```python
from build123d import *

# Parameters (mm, degrees)
F0_R     = 50
F1_DEPTH = 35
F2_R     = 25
F3_DEPTH = 35
F4_R     = 7
F5_DEPTH = 50.001


with BuildPart() as f1:
    # F0 (on Top) → F1 (new body)
    with BuildSketch(Plane.XY):
        Circle(F0_R)
    extrude(amount=F1_DEPTH)

    # F2 (on Top) → F3 (cut)
    with BuildSketch(Plane.XY):
        Circle(F2_R)
    extrude(amount=F3_DEPTH, mode=Mode.SUBTRACT)

    # F4 (on Right) → F5 (cut, through all)
    with BuildSketch(Plane.YZ):
        Circle(F4_R)
    extrude(amount=F5_DEPTH, mode=Mode.SUBTRACT)


solid = f1.part
```
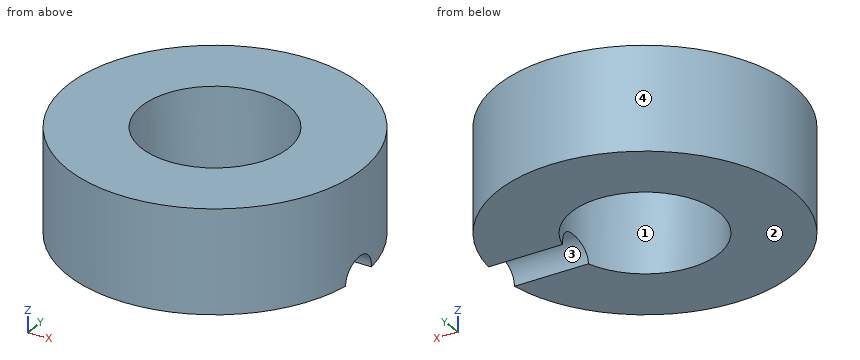
Build history of the part. All positions in model axes, mm. Face numbers are marked on the shaded views. Round coordinates to 2 decimals unless told otherwise and drop trailing zeros. Write each loop counter-clockwise with the first axis right and the second up, starting at its lowest first coordinate (ties: lowest second). Pieces come first, ordered by that corner, then holes.
1) Band-saw the part on B-B, the plane y = 0. List the corners of the cut face in (x, z).
2) Mould opens along Y. For the marked faces 1, 2, 3 and 4 say: +Y half, -Y half, draft (parallel to the pull), parting line (faces both ways), or undercut.
3) Band-saw the part on A-A, the plane x = 0. List the corners of the cut face in (y, z), and give its area (3 significant figures).
4) Drill centre lines: probe 1 along Y at (x, z) = (0, 26.5); probe 2 along Y at (x, z) = (-5, 33.5). Where is each one in solid material? Low to high.
5) Pin check, flat tips, straight feed: pin 1 (1 mm diameter, centred on x = 5, z = 10, fed in from -Y); pin 2 (1.5 mm diameter, centred on y = -34.5, z = 23.5, fed in from +X); pin 3 (8 mm diameter, centred on y = -25.5, z = 29.5, fed in from -X). Stop position of each tip, or through.
6) Band-saw the part on D-D, the plane y = -43. List the corners of the cut face in (x, z).
7) Band-saw the part on C-C, the plane z = 29.5. List the corners of the cut face in (x, y).
Ans:
1. outline: (-50, 0) - (-25, 0) - (-25, 35) - (-50, 35) - close; (25, 7) - (50, 7) - (50, 35) - (25, 35) - close
2. face 1: undercut
2. face 2: draft
2. face 3: undercut
2. face 4: parting line
3. outline: (-50, 0) - (-25, 0) - (-25, 35) - (-50, 35) - close; (25, 0) - (50, 0) - (50, 35) - (25, 35) - close
3. area: 1,750 mm2
4. probe 1: y = -50 to -25, 25 to 50
4. probe 2: y = -49.75 to -24.49, 24.49 to 49.75
5. pin 1: stops at y = -49.8
5. pin 2: stops at x = 36.89
5. pin 3: stops at x = -45.14
6. outline: (-25.51, 0) - (25.51, 0) - (25.51, 35) - (-25.51, 35) - close
7. outline: circle Ø100 at (0, 0); hole circle Ø50 at (0, 0)
